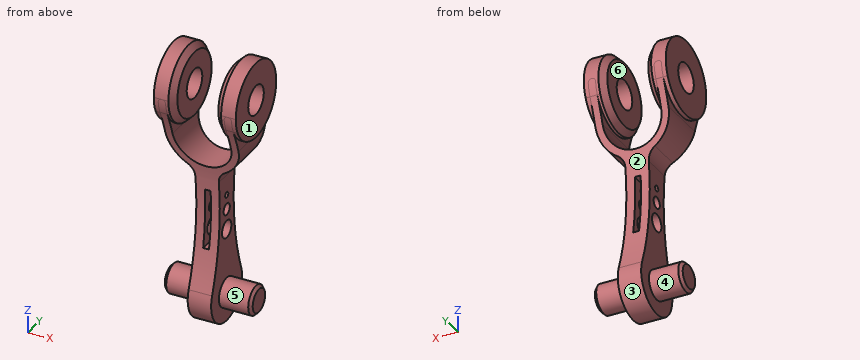
```python
from build123d import *

# Parameters (mm, degrees)
F1_DEPTH  = 19.05
F3_R      = 16.51
F4_DEPTH  = 17.78
F2_R      = 6.35
F6_DEPTH  = 38.1
F5_W      = 17.78
F5_H      = 38.1
F7_DEPTH  = 19.05
F8_SIZE   = 2.54
F10_DEPTH = 5.08
F11_R     = 6.35
F12_DEPTH = 19.05
F13_SIZE  = 1.27
F15_DEPTH = 38.1
F16_W     = 2.54
F16_H     = 25.4
F17_DEPTH = 25.4
F18_R     = 3.81
F18_R_2   = 2.54
F18_R_3   = 1.27
F19_DEPTH = 12.7
F20_ANGLE = 179.9946913403


with BuildPart() as f1:
    # F0 (on Front) → F1 (new body, symmetric)
    with BuildSketch(Plane.XZ):
        with BuildLine():
            ThreePointArc((-5.08, -13.9496366999), (-5.9049678847, -17.0795760164), (-8.1655181496, -19.3962556739))
            ThreePointArc((-8.1655181496, -19.3962556739), (-13.8198807904, -25.1910159629), (-15.8833905736, -33.02))
            Line((-15.8833905736, -33.02), (-15.8833905736, -49.276))
            ThreePointArc((-15.8833905736, -49.276), (-15.4370213081, -50.3536307345), (-14.3593905736, -50.8))
            Line((-14.3593905736, -50.8), (-14.224, -50.8))
            ThreePointArc((-14.224, -50.8), (-13.1463692655, -50.3536307345), (-12.7, -49.276))
            Line((-12.7, -49.276), (-12.7, -33.02))
            ThreePointArc((-12.7, -33.02), (0, -20.32), (12.7, -33.02))
            Line((12.7, -33.02), (12.7, -49.276))
            ThreePointArc((12.7, -49.276), (13.1463692655, -50.3536307345), (14.224, -50.8))
            Line((14.224, -50.8), (14.3593905736, -50.8))
            ThreePointArc((14.3593905736, -50.8), (15.4370213081, -50.3536307345), (15.8833905736, -49.276))
            Line((15.8833905736, -49.276), (15.8833905736, -33.02))
            ThreePointArc((15.8833905736, -33.02), (13.8198807904, -25.1910159629), (8.1655181496, -19.3962556739))
            ThreePointArc((8.1655181496, -19.3962556739), (5.9049678847, -17.0795760164), (5.08, -13.9496366999))
            Line((5.08, -13.9496366999), (5.08, 15.0491094791))
            Line((5.08, 15.0491094791), (-5.08, 15.0491094791))
            Line((-5.08, 15.0491094791), (-5.08, -13.9496366999))
        make_face()
    extrude(amount=F1_DEPTH, both=True)

    # F3 (on Right) → F4 (join, symmetric)
    with BuildSketch(Plane.YZ):
        with Locations((0, -50.8)):
            Circle(F3_R)
    extrude(amount=F4_DEPTH, both=True)

    # F2 (on Right) → F6 (cut, symmetric)
    with BuildSketch(Plane.YZ):
        with Locations((0, -50.8)):
            Circle(F2_R)
    extrude(amount=F6_DEPTH, both=True, mode=Mode.SUBTRACT)

    # F5 (on Front) → F7 (cut, symmetric)
    with BuildSketch(Plane.XZ):
        with Locations((0, -50.8)):
            Rectangle(F5_W, F5_H)
    extrude(amount=F7_DEPTH, both=True, mode=Mode.SUBTRACT)

    # F8
    f8_edges = [f1.edges().sort_by_distance(p)[0] for p in [
        (-8.89, -16.51, -50.8),
        (8.89, -16.51, -50.8),
    ]]
    chamfer(f8_edges, length=F8_SIZE)

    # F9 (on Right) → F10 (join, symmetric)
    with BuildSketch(Plane.YZ):
        with BuildLine():
            Line((19.0499954742, 12.6868685902), (19.0499954742, 38.0868685902))
            ThreePointArc((19.0499954742, 38.0868685902), (0, 57.15), (-19.0499954742, 38.0868685902))
            Line((-19.0499954742, 38.0868685902), (-19.0499954742, 12.6868685902))
            Line((-19.0499954742, 12.6868685902), (19.0499954742, 12.6868685902))
        make_face()
    extrude(amount=F10_DEPTH, both=True)

    # F11 (on Right) → F12 (join, symmetric)
    with BuildSketch(Plane.YZ):
        with Locations((0, 38.1)):
            Circle(F11_R)
    extrude(amount=F12_DEPTH, both=True)

    # F13
    f13_edges = [f1.edges().sort_by_distance(p)[0] for p in [
        (-19.05, -6.35, 38.1),
        (19.05, -6.35, 38.1),
    ]]
    chamfer(f13_edges, length=F13_SIZE)

    # F14 (on Right) → F15 (intersect, symmetric)
    with BuildSketch(Plane.YZ):
        with BuildLine():
            ThreePointArc((14.9945833541, -43.8904001536), (5.7486490124, -5.3934679933), (11.918771384, 33.714468254))
            ThreePointArc((11.918771384, 33.714468254), (0, 50.8), (-11.918771384, 33.714468254))
            ThreePointArc((-11.918771384, 33.714468254), (-5.7486490124, -5.3934679933), (-14.9945833541, -43.8904001536))
            ThreePointArc((-14.9945833541, -43.8904001536), (0, -67.31), (14.9945833541, -43.8904001536))
        make_face()
    extrude(amount=F15_DEPTH, both=True, mode=Mode.INTERSECT)

    # F16 (on Front) → F17 (cut, symmetric)
    with BuildSketch(Plane.XZ):
        with Locations((0, 3.8303633001)):
            Rectangle(F16_W, F16_H)
    extrude(amount=F17_DEPTH, both=True, mode=Mode.SUBTRACT)

    # F18 (on Right) → F19 (cut, symmetric)
    with BuildSketch(Plane.YZ):
        with Locations((0, 10.16)):
            Circle(F18_R)
        with Locations((0, 1.27)):
            Circle(F18_R_2)
        with Locations((0, -5.08)):
            Circle(F18_R_3)
    extrude(amount=F19_DEPTH, both=True, mode=Mode.SUBTRACT)


with BuildPart() as f1_1:
    # F20: moved
    add(f1.part.rotate(Axis((19.05, 0, 38.1), (1, 0, 0)), F20_ANGLE))


with BuildPart() as f1_2:
    # F22: moved
    add(f1_1.part.moved(Location((0, 0, -126.9999996184))))


solid = f1_2.part
```
Can you work these out from the model? Positions are in its coordinate system, mm. Face numbers are marked on the shaded views. A direction names the side the tool comes from. Give positions to 0.01 mm unless a question says otherwise; leave off trailing zeros. Loops run counter-clockwise (first coordinate to the right, second up) from the corner with the lowest first, then second, coordinate; pieces in that order, holes last. Notation, with made-up numbers: M 82,-29 L 106,-29 A19 cw 106,8 Z; hole C -40,35.5 d7. An arc over 180 degrees is marked long. Use one line per item in the form item = value. Start each with the question number.
(1) Please list where these lines run through material, in increasing order: line 1 (X direction, y = 9.5, z = -2); line 2 (X direction, y = -4.5, z = -65.5); line 3 (Z direction, x = 9, y = -2).
(2) I want a section at A-A, the plane x = 0. Write out the boundary of the cut face in (y, z), and give its area (3 significant figures).
(3) On a 3-axis mill with a long thin cutter (end or side, diameter ignored), from which of +Z, -Z, +X, -X, +Y, -Y can I reach the whole of each face in a straight line? I mean the marked faces 4, 5 and 6. Say none if no direction works.
(4) I'm going to push flat-ended pins straight in: P1, Ø6, axis at x = -12, y = -1, coming from the -Z side; P2, Ø4.5, axis at y = 2, z = -52.5, coming from the +X side; P3, Ø0.8, axis at x = -0.5, y = 1.5, coming from the +Z side; P4, Ø7.5, axis at y = 0.01, z = 0, coming from the -X side. Where does each tip first touch, or does it pass through?
(5) Thinking about a two-plate mould opening in Z: for the marked faces 1, 2 and 3, which applies, released by +Z, released by -Z, zero draft, split by the parting line, or undercut?
(6) I want a section at B-B, the plane x = 7. Write out the boundary of the cut face in (y, z), and give its area (3 significant figures).
(7) I want a section at C-C, the plane y = 0. State how many separate pieces and enclosed holes the cut face has, and give its area (3 significant figures).
Worked out:
q1.line_1 = -17.78 to -8.89, 8.89 to 17.78
q1.line_2 = -5.08 to -1.27, 1.27 to 5.08
q1.line_3 = -94.93 to -82.87, -30.87 to -26.74, -13.94 to -6.02, 6.02 to 13.94
q2.outline = M -11.92,-84.51 A12.7 ccw long 11.92,-84.52 A101.6 cw 7.26,-67.33 L -7.26,-67.33 A101.6 cw Z; M -7.45,-30.48 A101.6 cw -5.94,-41.93 L 5.95,-41.93 A101.6 cw 7.46,-30.48 Z
q2.area = 834 mm²
q3.face_4 = -X
q3.face_5 = +X
q3.face_6 = +Z, +Y, -Y
q4.P1 = -95.25
q4.P2 = 5.08
q4.P3 = -30.45
q4.P4 = through
q5.face_1 = zero draft
q5.face_2 = undercut
q5.face_3 = split by the parting line
q6.outline = M -7.87,-28.38 A101.6 cw -7.12,-32.3 L 7.13,-32.3 A101.6 cw 7.88,-28.38 Z; C 0,-88.9 d12.7
q6.area = 185 mm²
q7.separate_pieces = 8
q7.enclosed_holes = 0
q7.area = 1,370 mm²
